Could you check a few things on this model? Use its own coordinates, in mm. A direction names the side the tool comes from. Give positions to 0.01 mm unless a question says otherwise; leave off trailing zeros. Write each loop counter-clockwise with the first axis right and the second up, starting at its lowest first coordinate (ties: lowest second). Pieces come first, ordered by that corner, then holes. Notation, with made-up numbers: (-8, 39) - (8, 39) arc R37 ccw to (8, 78) - close; hole circle Ø3 at (-11, 49.25). An arc over 180 degrees is marked (long way). Answer in a Markdown table with one row per item.
from build123d import *

# Parameters (mm, degrees)
SKETCH1_R           = 12.5
BOSS_EXTRUDE1_DEPTH = 4
SKETCH2_R           = 5
CUT_EXTRUDE1_DEPTH  = 6
SKETCH3_R           = 2.25
CUT_EXTRUDE2_DEPTH  = 2


with BuildPart() as part:
    # Sketch1 → Boss-Extrude1 (new, symmetric)
    with BuildSketch(Plane.XY):
        Circle(SKETCH1_R)
    extrude(amount=BOSS_EXTRUDE1_DEPTH, both=True)

    # Sketch2 → Cut-Extrude1 (cut)
    with BuildSketch(Plane.XY.offset(4)):
        Circle(SKETCH2_R)
    extrude(amount=-CUT_EXTRUDE1_DEPTH, mode=Mode.SUBTRACT)

    # Sketch3 → Cut-Extrude2 (cut)
    with BuildSketch(Plane.XY.offset(-2)):
        Circle(SKETCH3_R)
    extrude(amount=-CUT_EXTRUDE2_DEPTH, mode=Mode.SUBTRACT)


solid = part.part
1) Imagine slicing it at D-D (x = -4.25). List the corners of the cut face in (y, z) for me, then the cut area to 3 significant figures.
Check values:
| item | result |
|---|---|
| outline | (-11.76, -4) - (11.76, -4) - (11.76, 4) - (2.63, 4) - (2.63, -2) - (-2.63, -2) - (-2.63, 4) - (-11.76, 4) - close |
| area | 156 mm2 |
2) We'd pull the mould along X, two halves only. Please class faces 3 (the face through (-0.29, 2.23, -2.99)), 4 (the face through (0, -3, -4)), 5 (the face through (11.923, 3.755, 0.056)): +X half, -X half, draft (parallel to the pull), parting line (faces both ways), or undercut.
Check values:
| item | result |
|---|---|
| face 3 | undercut |
| face 4 | draft |
| face 5 | parting line |
3) If I drill on line 1 (Y direction, x = 0, z = -2.4); line 2 (Y direction, x = 0, z = 1.9); line 3 (X direction, y = 0.25, z = -2.25), over which ranges is the centre line in solid material (lowest first)?
Check values:
| item | result |
|---|---|
| line 1 | y = -12.5 to -2.25, 2.25 to 12.5 |
| line 2 | y = -12.5 to -5, 5 to 12.5 |
| line 3 | x = -12.5 to -2.24, 2.24 to 12.5 |
4) Imagine slicing it at A-A (y = 0). List the corners of the cut face in (x, z) for me.
Check values:
| item | result |
|---|---|
| outline | (-12.5, -4) - (-2.25, -4) - (-2.25, -2) - (-5, -2) - (-5, 4) - (-12.5, 4) - close; (2.25, -4) - (12.5, -4) - (12.5, 4) - (5, 4) - (5, -2) - (2.25, -2) - close |
5) On a 3-axis mill with a long thin cutter (end or side, diameter ignored), from which of +Z, -Z, +X, -X, +Y, -Y can I reach the whole of each face in a straight line? I mean faces 1 (the face through (-0.2, -5.4, 4)), 2 (the face through (2.2, -1, -2)). Say none if no direction works.
Check values:
| item | result |
|---|---|
| face 1 | +Z, +X, -X, +Y, -Y |
| face 2 | +Z |
6) Will these pins go through, and if not, where does the flat tip stop? P1, Ø4, axis at x = -2.5, z = 1, coming from the +Y side; P2, Ø3, axis at y = 2.5, z = -0.5, coming from the +X side; P3, Ø2, axis at y = 3, z = 0.5, coming from the +X side; P4, Ø3.5, axis at x = 0, y = 0, coming from the +Z side.
Check values:
| item | result |
|---|---|
| P1 | stops at y = 12.49 |
| P2 | stops at x = 12.46 |
| P3 | stops at x = 12.34 |
| P4 | passes through |
7) Imagine slicing it at C-C (z = 0.75). List the corners of the cut face in (x, y) for me, then the cut area to 3 significant figures.
Check values:
| item | result |
|---|---|
| outline | circle Ø25 at (0, 0); hole circle Ø10 at (0, 0) |
| area | 412 mm2 |
